Input: dimensioned drawing with shaded views. Units: mm. Origin: part minimum x, y, z. Round coordinates to 2 decimals unless told otherwise and drop trailing zeros.
1) Ray query, line 1 along X through (y, z) = (2.5, 0.5); line 2 along X through (y, z) = (2.05, 5.5) (1 decimal); line 3 along X through (y, z) = (1.9, 9.75) (1 decimal). Return the intervals inside material, ascending.
2) Draft query along X for the marked faces 1, 2 and 3. Return one class per face: pulls with the +X half, pulls with the -X half, needs draft (parallel to the pull), parting line crosses it, or undercut.
3) First-contact query: pin 1 (1.4 mm diameter, centred on y = 0.5, z = 1, fed in from +X); pin 2 (1 mm diameter, centred on y = 2, z = 0.5, fed in from -X); pin 3 (1.5 mm diameter, centred on x = 14.5, z = 4, fed in from -Y). Flat tips, straight axial feed; report the tip coordinate or a pass-through.
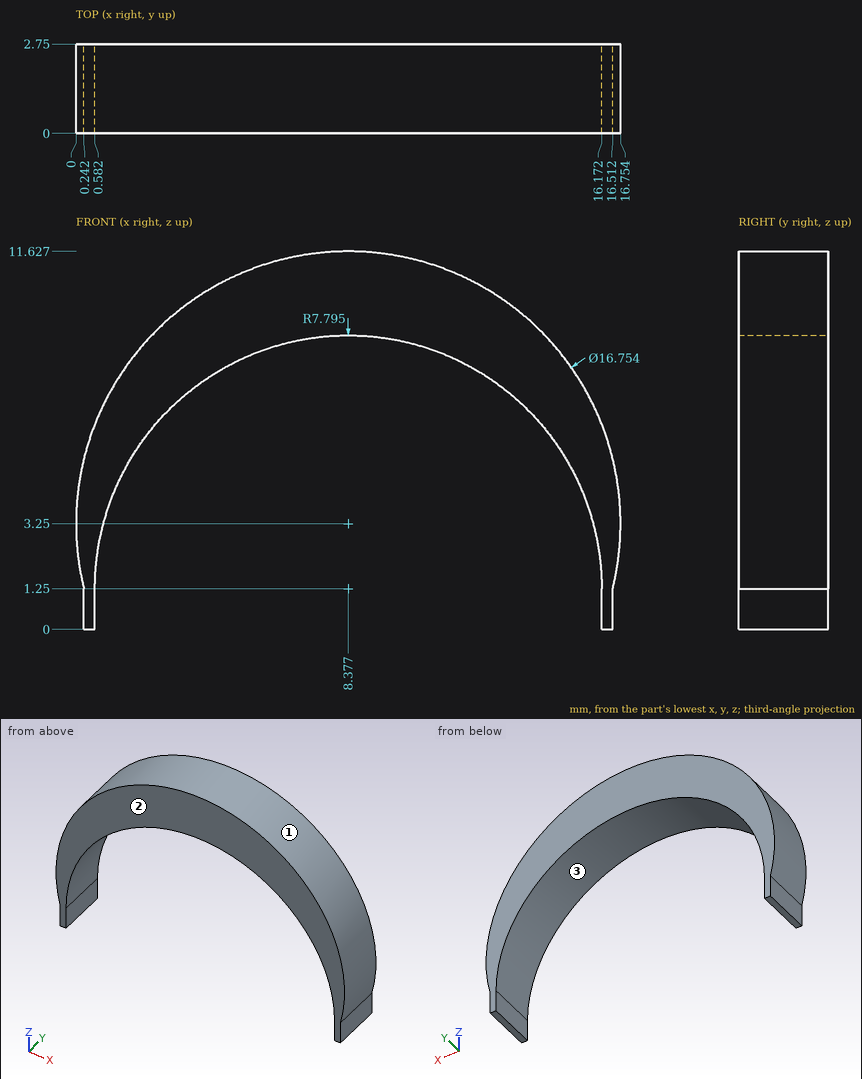
Final values:
1. line 1: x = 0.24 to 0.58, 16.17 to 16.51
1. line 2: x = 0.3 to 1.8, 14.9 to 16.4
1. line 3: x = 3.1 to 13.7
2. face 1: parting line crosses it
2. face 2: needs draft
2. face 3: undercut
3. pin 1: stops at x = 16.61
3. pin 2: stops at x = 0.24
3. pin 3: passes through
